```python
from build123d import *

# Parameters (mm, degrees)
F0_W     = 203.2
F0_H     = 152.4
F0_W_2   = 177.8
F0_H_2   = 127
F1_DEPTH = 6.35
F2_W     = 177.8
F2_H     = 127
F2_W_2   = 69.85
F2_H_2   = 44.45
F3_DEPTH = 3.175
F4_R     = 2.54
F5_DEPTH = 3.175
F6_R     = 2.54
F7_DEPTH = 2.54


with BuildPart() as f1:
    # F0 (on Top) → F1 (new body)
    with BuildSketch(Plane.XY):
        with Locations((101.6, 76.2)):
            Rectangle(F0_W, F0_H)
        with Locations((101.6, 76.2)):
            Rectangle(F0_W_2, F0_H_2, mode=Mode.SUBTRACT)
    extrude(amount=F1_DEPTH)

    # F2 (on Top) → F3 (join)
    with BuildSketch(Plane.XY):
        with Locations((101.6, 76.2)):
            Rectangle(F2_W, F2_H)
        with Locations((60.325, 47.625)):
            Rectangle(F2_W_2, F2_H_2, mode=Mode.SUBTRACT)
        with Locations((142.875, 47.625)):
            Rectangle(F2_W_2, F2_H_2, mode=Mode.SUBTRACT)
        with Locations((60.325, 104.775)):
            Rectangle(F2_W_2, F2_H_2, mode=Mode.SUBTRACT)
        with Locations((142.875, 104.775)):
            Rectangle(F2_W_2, F2_H_2, mode=Mode.SUBTRACT)
    extrude(amount=F3_DEPTH)

    # F4 (on face) → F5 (join, through all)
    with BuildSketch(Plane.XY.offset(3.175)):
        with Locations((19.05, 133.35)):
            Circle(F4_R)
        with Locations((19.05, 19.05)):
            Circle(F4_R)
        with Locations((184.15, 19.05)):
            Circle(F4_R)
    extrude(amount=F5_DEPTH)

    # F6 (on face) → F7 (cut)
    with BuildSketch(Plane.XY.offset(3.175)):
        with Locations((60.325, 133.35)):
            Circle(F6_R)
        with Locations((142.875, 133.35)):
            Circle(F6_R)
        with Locations((101.6, 47.625)):
            Circle(F6_R)
        with Locations((101.6, 104.775)):
            Circle(F6_R)
        with Locations((142.875, 76.2)):
            Circle(F6_R)
        with Locations((60.325, 19.05)):
            Circle(F6_R)
        with Locations((184.15, 47.625)):
            Circle(F6_R)
        with Locations((142.875, 19.05)):
            Circle(F6_R)
        with Locations((19.05, 47.625)):
            Circle(F6_R)
        with Locations((184.15, 104.775)):
            Circle(F6_R)
        with Locations((60.325, 76.2)):
            Circle(F6_R)
        with Locations((19.05, 104.775)):
            Circle(F6_R)
    extrude(amount=-F7_DEPTH, mode=Mode.SUBTRACT)


solid = f1.part
```
Build history of the part. All positions in model axes, mm. A direction names the side the tool comes from. Give positions to 0.01 mm unless a question says otherwise; leave off trailing zeros. Loops run counter-clockwise (first coordinate to the right, second up) from the corner with the lowest first, then second, coordinate; pieces in that order, holes last.
1) Two-plate mould, pull along Y, no slides. Class faces 1 (the face through (184, 19, 6.35)), 2 (the face through (100, 77, 3.175)), 3 (the face through (100, 0, 3)), 4 (the face through (100, 152.4, 3)): released by +Y, released by -Y, zero draft, split by the parting line, or undercut.
Values follow:
face 1: zero draft
face 2: undercut
face 3: released by -Y
face 4: released by +Y
2) Probe line 1 along Y through (x, z) = (184.15, 1.8) (3 decimals); line 2 along Y through (x, z) = (125.5, 2.5); line 3 along X through (y, z) = (92.5, 2.25). List the from-to ranges inside material, lowest first.
Values follow:
line 1: y = 0 to 45.085, 50.165 to 102.235, 107.315 to 152.4
line 2: y = 0 to 25.4, 69.85 to 82.55, 127 to 152.4
line 3: x = 0 to 25.4, 95.25 to 107.95, 177.8 to 203.2
3) 3-axis set-ups, long thin cutter, end or side, ignore diameter. For faces 5 (the face through (19, 19, 6.35)), 6 (the face through (184, 48, 0.635)): which of +Z, -Z, +X, -X, +Y, -Y reach the whole face in a straight line?
Values follow:
face 5: +Z, +X, -X, +Y, -Y
face 6: +Z
4) Band-saw the part on B-B on y = 65.5. List the corners of the cut face in (x, z) (3 decimals), then the cut area to 3 significant figures.
Values follow:
outline: (0, 0) - (25.4, 0) - (25.4, 3.175) - (12.7, 3.175) - (12.7, 6.35) - (0, 6.35) - close; (95.25, 0) - (107.95, 0) - (107.95, 3.175) - (95.25, 3.175) - close; (177.8, 0) - (203.2, 0) - (203.2, 6.35) - (190.5, 6.35) - (190.5, 3.175) - (177.8, 3.175) - close
area: 282 mm2
5) Band-saw the part on D-D on x = 184.15. List the corners of the cut face in (y, z) (3 decimals), then the cut area to 3 significant figures.
Values follow:
outline: (0, 0) - (152.4, 0) - (152.4, 6.35) - (139.7, 6.35) - (139.7, 3.175) - (107.315, 3.175) - (107.315, 0.635) - (102.235, 0.635) - (102.235, 3.175) - (50.165, 3.175) - (50.165, 0.635) - (45.085, 0.635) - (45.085, 3.175) - (21.59, 3.175) - (21.59, 6.35) - (16.51, 6.35) - (16.51, 3.175) - (12.7, 3.175) - (12.7, 6.35) - (0, 6.35) - close
area: 555 mm2
6) Drop flat-ended pins along their axis: P1, Ø6, axis at x = 101.6, y = 47.625, coming from the +Z side (3 decimals); P2, Ø2.5, axis at x = 102.5, y = 47, coming from the +Z side (3 decimals). Give the stop position or say it passes through.
Values follow:
P1: stops at z = 3.175
P2: stops at z = 0.635
7) Band-saw the part on C-C on x = 135. List the corners of the cut face in (y, z) (3 decimals).
Values follow:
outline: (0, 0) - (25.4, 0) - (25.4, 3.175) - (12.7, 3.175) - (12.7, 6.35) - (0, 6.35) - close; (69.85, 0) - (82.55, 0) - (82.55, 3.175) - (69.85, 3.175) - close; (127, 0) - (152.4, 0) - (152.4, 6.35) - (139.7, 6.35) - (139.7, 3.175) - (127, 3.175) - close
8) Band-saw the part on A-A on z = 4.5. List the corners of the cut face in (x, y).
Values follow:
outline: (0, 0) - (203.2, 0) - (203.2, 152.4) - (0, 152.4) - close; circle Ø5.08 at (19.05, 19.05); circle Ø5.08 at (19.05, 133.35); circle Ø5.08 at (184.15, 19.05); hole (12.7, 12.7) - (190.5, 12.7) - (190.5, 139.7) - (12.7, 139.7) - close
